Design review of the part built by this model. Coordinates are the model's own, in mm. A direction names the side the tool comes from. Give positions to 0.01 mm unless a question says otherwise; leave off trailing zeros. Order: outer loops, then holes, each group sorted by start corner. A loop starts at its lowest first (then second) coordinate and runs counter-clockwise, first axis right, second up. Notation, with made-up numbers: (23.25, -39.5) -> (52.25, -39.5) arc R14 cw to (52.25, -12.5) -> close; hole circle Ø11 at (80, -27.5). An arc over 180 degrees is marked (long way). One line per item, written item: value.
from build123d import *

# Parameters (mm, degrees)
F0_W     = 228.6
F0_H     = 152.4
F1_DEPTH = 203.2
F2_W     = 127
F2_H     = 50.8
F3_DEPTH = 127
F5_DEPTH = 101.6


# Not quite as in the source:
# - a feature names something its author has since deleted; it is built from what else it names


with BuildPart() as f1:
    # F0 (on Top) → F1 (new body)
    with BuildSketch(Plane.XY):
        with Locations((10.0263133645, -15.0303587328)):
            Rectangle(F0_W, F0_H)
    extrude(amount=F1_DEPTH)

    # F2 (on face) → F3 (cut)
    with BuildSketch(Plane.XY.offset(203.2)):
        with Locations((60.8263133645, -65.8303587328)):
            Rectangle(F2_W, F2_H)
    extrude(amount=-F3_DEPTH, mode=Mode.SUBTRACT)

    # F4 (on face) → F5 (cut)
    with BuildSketch(Plane.XZ.offset(40.4303587328)):
        Polygon((124.3263133645, 203.2), (48.1263133645, 203.2), (124.3263133645, 127), align=None)
    extrude(amount=-F5_DEPTH, mode=Mode.SUBTRACT)


solid = f1.part
Item 1: Add section B-B on x = 43. Give the boundary of the cut face in (y, z).
Returned:
outline: (-91.23, 0) -> (61.17, 0) -> (61.17, 203.2) -> (-40.43, 203.2) -> (-40.43, 76.2) -> (-91.23, 76.2) -> close
Item 2: Machinability: for faces 1 (the flat face through (-29, -14, 203.2)), 2 (the flat face through (-2.674, -66, 141)), which of the approach directions +Z, -Z, +X, -X, +Y, -Y give a long, thin tool a straight path to every point of the face, cutting with its end or side? Answer none if there is none.
Returned:
face 1: +Z, +X, -X, +Y, -Y
face 2: +Z, +X, -Y
Item 3: Add section A-A on y = -52.5. Give the boundary of the cut face in (x, z).
Returned:
outline: (-104.27, 0) -> (124.33, 0) -> (124.33, 76.2) -> (-2.67, 76.2) -> (-2.67, 203.2) -> (-104.27, 203.2) -> close
Item 4: Clearance check with flat-ended pins moving along their axes: P1, Ø4, axis at x = -60.5, y = -52, coming from the -Z side; P2, Ø2, axis at x = 16.5, y = -66, coming from the +Z side; P3, Ø5, axis at y = -55, z = 169, coming from the +X side. State where each tip first meets the part, or that it passes through.
Returned:
P1: z = 0
P2: z = 76.2
P3: x = -2.67
Item 5: To check wall thickness, follow line 1 along X through (y, z) = (-49.5, 97); line 2 along Z through (x, y) = (57, -55.5); line 3 along Y through (x, z) = (5.5, 145.5). State the ranges of each line that lie inside material, in increasing order. Write a range as from..to.
Returned:
line 1: -104.27..-2.67
line 2: 0..76.2
line 3: -40.43..61.17
Item 6: Add section C-C on y = 8. Give the boundary of the cut face in (x, z), plus the area to 3 significant figures.
Returned:
outline: (-104.27, 0) -> (124.33, 0) -> (124.33, 127) -> (48.13, 203.2) -> (-104.27, 203.2) -> close
area: 43,500 mm²
